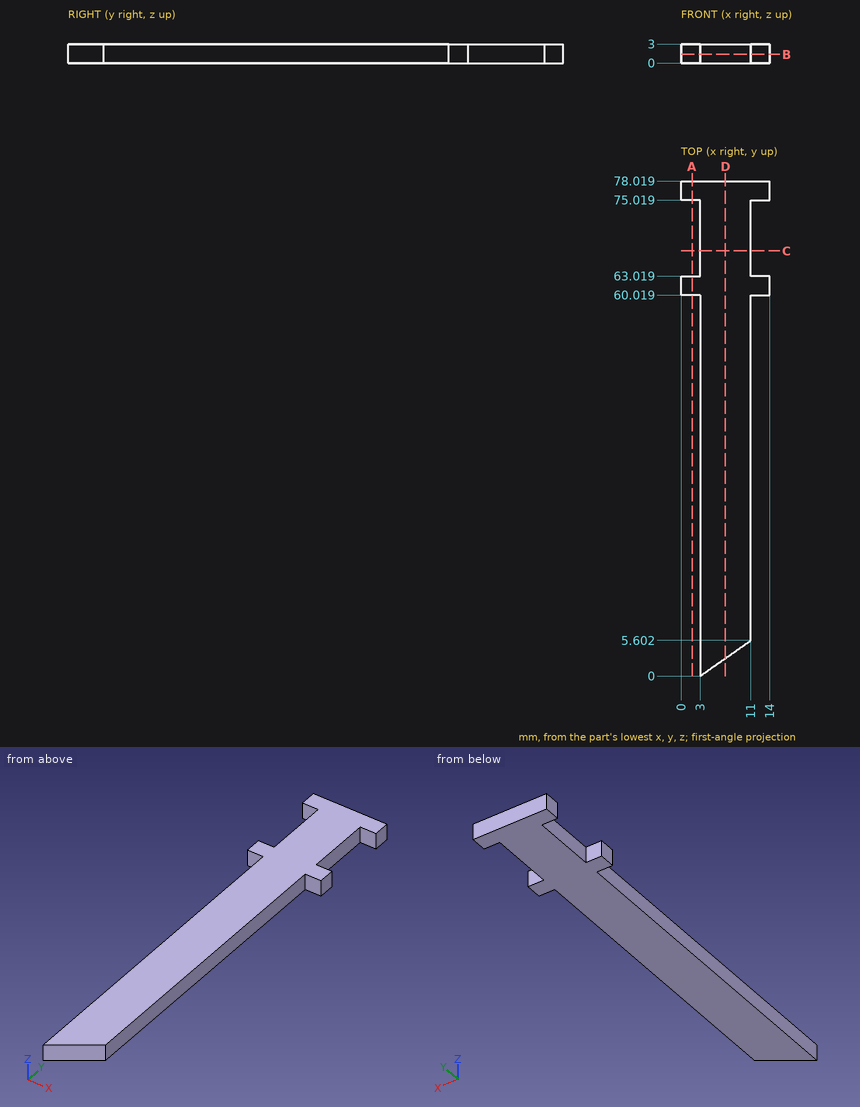
Input: dimensioned drawing with shaded views. Units: mm. Origin: part minimum x, y, z. Round coordinates to 2 decimals unless told otherwise and drop trailing zeros. Loops run counter-clockwise (first coordinate to the right, second up) from the corner with the lowest first, then second, coordinate; pieces in that order, holes last. Notation, with made-up numbers: M -1,76.5 L 35,76.5 A23 cw 35,96.5 Z; hole C -32.75,34 d1. An arc over 180 degrees is marked long. Return JSON: item names as keys, results as strings. Group by question number.
1. Section query A-A on x = 1.75. Output: boundary loops of the cut face in (y, z).
2. Pin query (flat end, axial travel): pin 1 (1 mm diameter, centred on x = 10, z = 1, fed in from -Y); pin 2 (0.9 mm diameter, centred on y = 45.5, z = 1, fed in from +X); pin 3 (0.9 mm diameter, centred on x = 13, z = 2, fed in from -Y). Return the tip coordinate at first contact, or that it passes through.
3. Section query B-B on z = 1.35. Output: boundary loops of the cut face in (x, y).
4. Section query C-C on y = 67. Output: boundary loops of the cut face in (x, z), and give its area (3 significant figures).
5. Material intervals for line 1 along Y through (x, z) = (2, 1.4); line 2 along X through (y, z) = (44, 2.3); line 3 along Y through (x, z) = (10.75, 2.3), sorted ascending. Write a range as from..to.
6. Section query D-D on x = 7. Output: boundary loops of the cut face in (y, z).
Checks:
{
 "1": {"outline": "M 60.02,0 L 63.02,0 L 63.02,3 L 60.02,3 Z; M 75.02,0 L 78.02,0 L 78.02,3 L 75.02,3 Z"},
 "2": {"pin 1": "stops at y = 4.55", "pin 2": "stops at x = 11", "pin 3": "stops at y = 60.02"},
 "3": {"outline": "M 0,60.02 L 3,60.02 L 3,0 L 11,5.6 L 11,60.02 L 14,60.02 L 14,63.02 L 11,63.02 L 11,75.02 L 14,75.02 L 14,78.02 L 0,78.02 L 0,75.02 L 3,75.02 L 3,63.02 L 0,63.02 Z"},
 "4": {"outline": "M 3,0 L 11,0 L 11,3 L 3,3 Z", "area": "24.0 mm²"},
 "5": {"line 1": "y = 60.02..63.02, 75.02..78.02", "line 2": "x = 3..11", "line 3": "y = 5.43..78.02"},
 "6": {"outline": "M 2.8,0 L 78.02,0 L 78.02,3 L 2.8,3 Z"}
}
